from build123d import *

# Parameters (mm, degrees)
SKETCH1_R           = 2.794
SKETCH1_R_2         = 3.175
BOSS_EXTRUDE1_DEPTH = 6.35


with BuildPart() as part:
    # Sketch1 → Boss-Extrude1 (new body)
    with BuildSketch(Plane(origin=(0, 0, 0), x_dir=(0, 0, -1), z_dir=(1, 0, 0))):
        with BuildLine():
            Line((2.573887506, 9.828565669), (-70.482178955, 28.960359974))
            ThreePointArc((-70.482178955, 28.960359974), (-75.490460705, -10.374504448), (-60.056829366, -46.900077255))
            Line((-60.056829366, -46.900077255), (5.129832124, -8.769858743))
            ThreePointArc((5.129832124, -8.769858743), (10.065394761, 1.38326726), (2.573887506, 9.828565669))
        make_face()
        with Locations((-33.347167041, 10.699986838)):
            Circle(SKETCH1_R, mode=Mode.SUBTRACT)
        with Locations((-33.832816449, 3.25056569)):
            Circle(SKETCH1_R, mode=Mode.SUBTRACT)
        with Locations((-33.276980509, -4.193947538)):
            Circle(SKETCH1_R, mode=Mode.SUBTRACT)
        with Locations((-31.690477935, -11.488653864)):
            Circle(SKETCH1_R, mode=Mode.SUBTRACT)
        with Locations((-29.104188196, -18.491570126)):
            Circle(SKETCH1_R, mode=Mode.SUBTRACT)
        Circle(SKETCH1_R_2, mode=Mode.SUBTRACT)
    extrude(amount=BOSS_EXTRUDE1_DEPTH)


solid = part.part
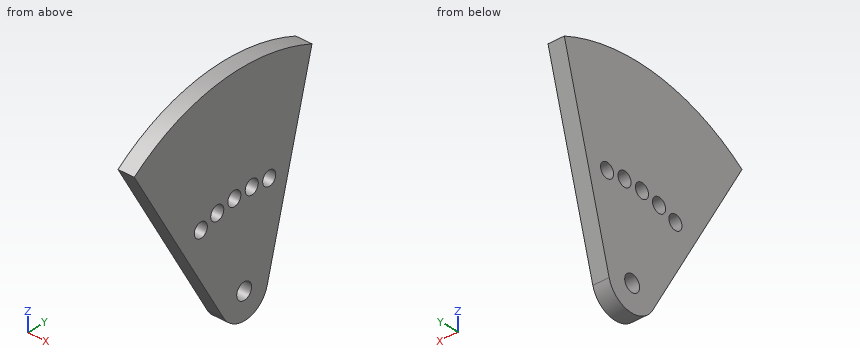
The listing builds one solid part. Answer for the finished solid, in the listing's coordinates (mm). Coordinates: 2 decimals unless noted, no trailing zeros. Write each loop counter-clockwise with the first axis right and the second up, starting at its lowest first coordinate (ties: lowest second). Pieces come first, ordered by that corner, then holes. Notation, with made-up numbers: (11, -38) - (28, -38) arc R16 cw to (28, -22) - close; hole circle Ø1 at (24, 84). An arc over 180 degrees is marked (long way). Answer as CSV lines item,"result".
1. Find section C-C (x = 4). Give the vertices of the cut face in (y, z) (3 decimals).
Computed values:
outline,"(-46.9, 60.057) - (-8.77, -5.13) arc R10.16 ccw to (9.829, -2.574) - (28.96, 70.482) arc R76.2 ccw to start; hole circle Ø5.588 at (-18.492, 29.104); hole circle Ø5.588 at (-11.489, 31.69); hole circle Ø5.588 at (-4.194, 33.277); hole circle Ø6.35 at (0, 0); hole circle Ø5.588 at (3.251, 33.833); hole circle Ø5.588 at (10.7, 33.347)"
2. Given P1, Ø1, axis at x = 4, z = 36.5, coming from the +Y side; P2, Ø9, axis at y = -4.19, z = 33.28, coming from the +X side; P3, Ø1, axis at x = 3.5, z = 5, coming from the -Y side, each flat-ended and moving along its own axis, determine where each tip first touches the part or whether it passes through.
Computed values:
P1,"stops at y = 20.19"
P2,"stops at x = 6.35"
P3,"stops at y = -14.99"
3. Straight lines are drawn through the part: line 1 (Y direction, x = 1.75, z = 31); line 2 (Z direction, x = 3, y = 2); line 3 (Z direction, x = 4.25, y = 4). For each, find the intervals that lie inside material, in ascending order. Write a range as [from, to].
Computed values:
line 1,"y = [-29.9, -20.54], [-16.44, -14.2], [-8.78, -5.81], [-2.57, 9.18], [12.22, 18.62]"
line 2,"z = [-9.96, -2.47], [2.47, 31.33], [36.33, 76.17]"
line 3,"z = [-9.34, 31.14], [36.52, 76.09]"
4. Find section D-D (z = 66.5). Give the vertices of the cut face in (x, y), plus the area to 3 significant figures.
Computed values:
outline,"(0, -37.2) - (6.35, -37.2) - (6.35, 27.92) - (0, 27.92) - close"
area,"414 mm²"
5. Find section A-A (y = -10.5). Give the vertices of the cut face in (x, z), plus the area to 3 significant figures.
Computed values:
outline,"(0, -2.17) - (6.35, -2.17) - (6.35, 29.08) - (0, 29.08) - close; (0, 34.3) - (6.35, 34.3) - (6.35, 75.47) - (0, 75.47) - close"
area,"460 mm²"
